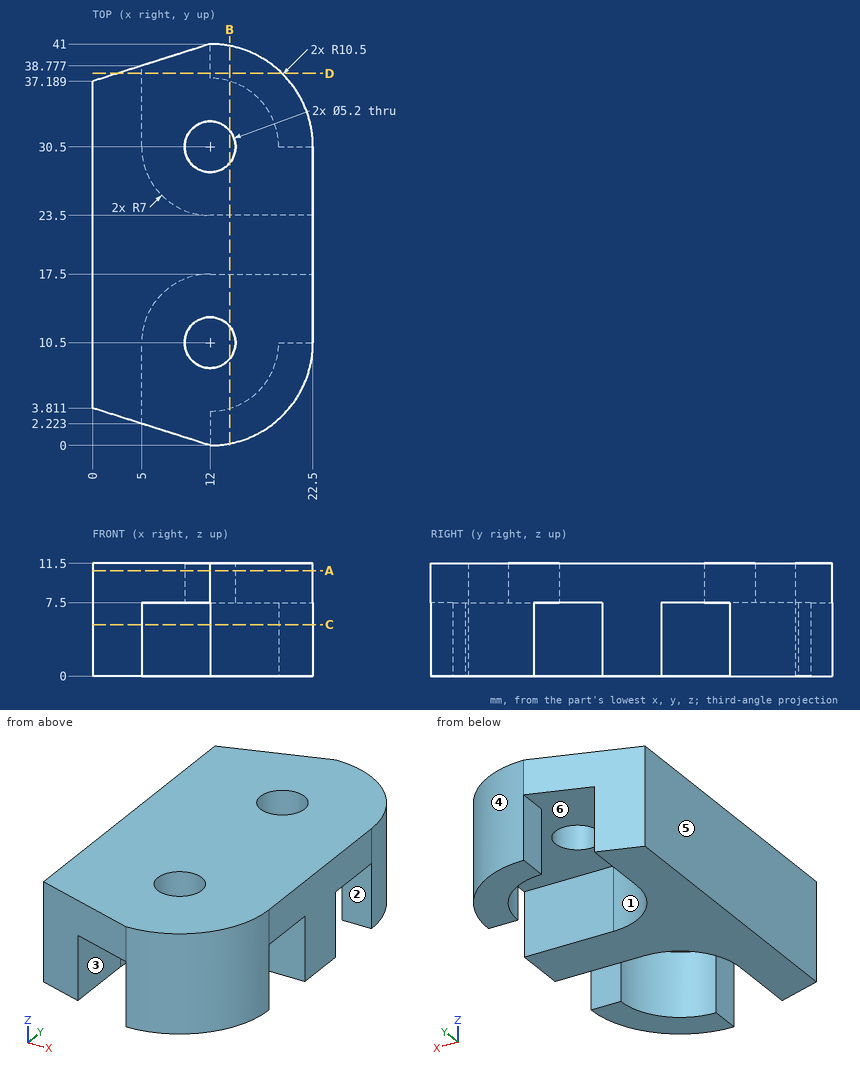
Part print with two shaded views. Sizes in mm from the minimum x, y, z corner. A direction names the side the tool comes from. Round coordinates to 2 decimals unless told otherwise and drop trailing zeros. Order: outer loops, then holes, each group sorted by start corner. A loop starts at its lowest first (then second) coordinate and runs counter-clockwise, first axis right, second up. Notation, with made-up numbers: (46.5, 67.25) - (50.5, 67.25) arc R19 cw to (50.5, 99.25) - close; hole circle Ø4 at (10.25, 24). An arc over 180 degrees is marked (long way). Answer in a Markdown table with one row per item. Add a question column.
(1) 3-axis set-ups, long thin cutter, end or side, ignore diameter. For the marked faces 1, 2 and 3: which of +Z, -Z, +X, -X, +Y, -Y reach the whole face in a straight line?
(2) Drop flat-ended pins along their axis: pin 1 Ø3 at (x, z) = (21, 4) entering from -Y; pin 2 Ø1.8 at (y, z) = (40, 3.5) entering from -X; pin 3 Ø3 at (x, z) = (3.5, 8) entering from +Y. Give the stop position or say it passes through.
(3) Band-saw the part on D-D on y = 38. List the corners of the cut face in (x, z), and give its area (3 significant figures).
(4) Band-saw the part on C-C on z = 5.25. List the corners of the cut face in (x, y).
(5) Band-saw the part on A-A on z = 10.75. List the corners of the cut face in (x, y), and give its area (3 significant figures).
(6) Band-saw the part on B-B on x = 14. List the corners of the cut face in (y, z).
(7) Probe L1, parallel to X at y = 10.5, z = 8.4; L2, parallel to Y at x = 10, z = 11 (1 decimal); L3, parallel to Y at x = 19.5, z = 0.75. List the from-to ranges inside material, lowest first. Write a range as [from, to].
(8) Mould opens along Y. For the marked faces 4, 5 and 6 say: +Y half, -Y half, draft (parallel to the pull), parting line (faces both ways), or undercut.
Data:
| question | item | result |
|---|---|---|
| 1 | face 1 | -Z, +X, +Y |
| 1 | face 2 | -Z, +X |
| 1 | face 3 | -Z, -Y |
| 2 | pin 1 | stops at y = 3.15 |
| 2 | pin 2 | stops at x = 12 |
| 2 | pin 3 | stops at y = 38.78 |
| 3 | outline | (2.55, 0) - (5, 0) - (5, 7.5) - (12, 7.5) - (12, 0) - (19.35, 0) - (19.35, 11.5) - (2.55, 11.5) - close |
| 3 | area | 141 mm^2 |
| 4 | outline | (0, 3.81) - (5, 2.22) - (5, 10.5) arc R7 cw to (12, 17.5) - (22.5, 17.5) - (22.5, 23.5) - (12, 23.5) arc R7 cw to (5, 30.5) - (5, 38.78) - (0, 37.19) - close; (12, 0) arc R10.5 ccw to (22.5, 10.5) - (19, 10.5) arc R7 cw to (12, 3.5) - close; (12, 37.5) arc R7 cw to (19, 30.5) - (22.5, 30.5) arc R10.5 ccw to (12, 41) - close |
| 5 | outline | (0, 3.81) - (12, 0) arc R10.5 ccw to (22.5, 10.5) - (22.5, 30.5) arc R10.5 ccw to (12, 41) - (0, 37.19) - close; hole circle Ø5.2 at (12, 10.5); hole circle Ø5.2 at (12, 30.5) |
| 5 | area | 787 mm^2 |
| 6 | outline | (0.19, 0) - (3.79, 0) - (3.79, 7.5) - (8.84, 7.5) - (8.84, 11.5) - (0.19, 11.5) - close; (12.16, 7.5) - (17.5, 7.5) - (17.5, 0) - (23.5, 0) - (23.5, 7.5) - (28.84, 7.5) - (28.84, 11.5) - (12.16, 11.5) - close; (32.16, 7.5) - (37.21, 7.5) - (37.21, 0) - (40.81, 0) - (40.81, 11.5) - (32.16, 11.5) - close |
| 7 | L1 | x = [0, 9.4], [14.6, 22.5] |
| 7 | L2 | y = [0.6, 8.8], [12.2, 28.8], [32.2, 40.4] |
| 7 | L3 | y = [3.15, 10.5], [17.5, 23.5], [30.5, 37.85] |
| 8 | face 4 | +Y half |
| 8 | face 5 | draft |
| 8 | face 6 | undercut |
